Part model, mm, in its own coordinate system. A direction names the side the tool comes from. Round coordinates to 2 decimals unless told otherwise and drop trailing zeros. Loops run counter-clockwise (first coordinate to the right, second up) from the corner with the lowest first, then second, coordinate; pieces in that order, holes last. Notation, with made-up numbers: M 70,-37 L 88,-37 A19 ccw 88,-32 Z; hole C -22.5,60.5 d11. An arc over 180 degrees is marked long. Put each result on its own line as item: value. Start each with the question number.
1) Slice it at C-C on z = -5.92. State how many separate pieces and enclosed holes the cut face has, then the cut area to 3 significant figures.
2) Probe line 1 along Z through (x, y) = (6.35, 2.35) (3 decimals); line 2 along X through (y, z) = (33.5, 7.5) (3 decimals); line 3 along Y through (x, z) = (-8, -0.5) (3 decimals). List the from-to ranges inside material, lowest first.
3) Which spindle directions (+Z, -Z, +X, -X, +Y, -Y) get a long thin tool onto all of the face, cutting with end or side? Do faces 5 (the flat face through (22.225, 25, 0)), 6 (the cylindrical face through (23.835, 14.274, -5.713)). Say none if no direction does.
4) Slice it at A-A on y = 31.75. Give the cut face in (x, z) (1 decimal).
5) Drop a flat-ended pin along its axis: pin 1 Ø8.5 at (x, z) = (6.35, 0) entering from +Y (3 decimals). Give the stop position or say it passes through.
6) Slice it at B-B on x = 6.35. Give the cut face in (y, z) (3 decimals), then the cut area to 3 significant figures.
7) Pull direction X, two halves, no side cores. Call faces 1 (the flat face through (-25.4, 2, 0)), 2 (the flat face through (11, 3, 11)), 3 (the flat face through (25.4, 22, 0)), 4 (the cylindrical face through (3.18, 1.57, 0.14)): +X half, -X half, draft (parallel to the pull), parting line (faces both ways), or undercut.
```python
from build123d import *

# Parameters (mm, degrees)
BOSS_EXTRUDE1_DEPTH = 11
FILLET1_R           = 1.5875
SKETCH3_W           = 24.423912887
SKETCH3_H           = 26.552361768
CUT_EXTRUDE1_DEPTH  = 23
SKETCH4_R           = 3.175
CUT_EXTRUDE2_DEPTH  = 45.45
SKETCH5_R           = 1.5875
CUT_EXTRUDE3_DEPTH  = 51.8


with BuildPart() as part:
    # Sketch2 → Boss-Extrude1 (new body, symmetric)
    with BuildSketch(Plane.XY):
        Polygon((-25.4, 0), (25.4, 0), (25.4, 50.8), (22.225, 50.8), (22.225, 3.175), (-25.4, 3.175), align=None)
    extrude(amount=BOSS_EXTRUDE1_DEPTH, both=True)

    # Fillet1
    fillet1_edges = [part.edges().sort_by_distance(p)[0] for p in [
        (22.225, 3.175, 0),
    ]]
    fillet(fillet1_edges, radius=FILLET1_R)

    # Sketch3 → Cut-Extrude1 (cut, through all)
    with BuildSketch(Plane.XY.offset(11)):
        with Locations((18.271034128, 57.726180884)):
            Rectangle(SKETCH3_W, SKETCH3_H)
    extrude(amount=-CUT_EXTRUDE1_DEPTH, mode=Mode.SUBTRACT)

    # Sketch4 → Cut-Extrude2 (cut, through all)
    with BuildSketch(Plane.XZ):
        with Locations((-12.7, 0)):
            Circle(SKETCH4_R)
        with Locations((6.35, 0)):
            Circle(SKETCH4_R)
    extrude(amount=-CUT_EXTRUDE2_DEPTH, mode=Mode.SUBTRACT)

    # Sketch5 → Cut-Extrude3 (cut, through all)
    with BuildSketch(Plane(origin=(25.4, 0, 0), x_dir=(0, 0, -1), z_dir=(1, 0, 0))):
        with Locations((5.92, 31.75)):
            Circle(SKETCH5_R)
        with Locations((5.92, 12.7)):
            Circle(SKETCH5_R)
    extrude(amount=-CUT_EXTRUDE3_DEPTH, mode=Mode.SUBTRACT)


solid = part.part
```
Recorded:
1. separate pieces: 3
1. enclosed holes: 0
1. area: 273 mm2
2. line 1: z = -11 to -3.175, 3.175 to 11
2. line 2: x = 22.225 to 25.4
2. line 3: y = 0 to 3.175
3. face 5: +Z, -Z, -X, +Y
3. face 6: +X, -X
4. outline: M 22.2,-11 L 25.4,-11 L 25.4,-7.5 L 22.2,-7.5 Z; M 22.2,-4.3 L 25.4,-4.3 L 25.4,11 L 22.2,11 Z
5. pin 1: stops at y = 3.175
6. outline: M 0,-11 L 3.175,-11 L 3.175,-3.175 L 0,-3.175 Z; M 0,3.175 L 3.175,3.175 L 3.175,11 L 0,11 Z
6. area: 49.7 mm2
7. face 1: -X half
7. face 2: draft
7. face 3: +X half
7. face 4: undercut
